from build123d import *

# Parameters (mm, degrees)
SKETCH1_W           = 50
SKETCH1_H           = 100
SKETCH1_R           = 2
SKETCH1_R_2         = 2.5
SKETCH1_W_2         = 3
SKETCH1_H_2         = 20
BOSS_EXTRUDE1_DEPTH = 3
SKETCH2_W           = 3
SKETCH2_H           = 10
CUT_EXTRUDE1_DEPTH  = 10
SKETCH3_W           = 5
SKETCH3_H           = 3
CUT_EXTRUDE2_DEPTH  = 56.982140009


with BuildPart() as part:
    # Sketch1 → Boss-Extrude1 (new body)
    with BuildSketch(Plane.XY):
        Rectangle(SKETCH1_W, SKETCH1_H)
        with Locations((-9, 44)):
            Circle(SKETCH1_R, mode=Mode.SUBTRACT)
        with Locations(Location((9, 44, 0), (0, 0, 180))):
            Circle(SKETCH1_R, mode=Mode.SUBTRACT)
        with Locations(Location((-9, 20, 0), (0, 0, 180))):
            Circle(SKETCH1_R, mode=Mode.SUBTRACT)
        with Locations((9, 20)):
            Circle(SKETCH1_R, mode=Mode.SUBTRACT)
        with Locations((-7.5, -45)):
            Circle(SKETCH1_R_2, mode=Mode.SUBTRACT)
        with Locations(Location((7.5, -45, 0), (0, 0, 180))):
            Circle(SKETCH1_R_2, mode=Mode.SUBTRACT)
        with Locations((6, -6.851771234)):
            Rectangle(SKETCH1_W_2, SKETCH1_H_2, mode=Mode.SUBTRACT)
        with Locations((-6, -6.851771234)):
            Rectangle(SKETCH1_W_2, SKETCH1_H_2, mode=Mode.SUBTRACT)
    extrude(amount=BOSS_EXTRUDE1_DEPTH)

    # Sketch2 → Cut-Extrude1 (cut)
    with BuildSketch(Plane.XY.offset(3)):
        with Locations((3.25, -25)):
            Rectangle(SKETCH2_W, SKETCH2_H)
        with Locations((-3.25, -25)):
            Rectangle(SKETCH2_W, SKETCH2_H)
    extrude(amount=-CUT_EXTRUDE1_DEPTH, mode=Mode.SUBTRACT)

    # Sketch3 → Cut-Extrude2 (cut, through all)
    with BuildSketch(Plane.XY.offset(3)):
        with Locations((-7.5, -34.709613659)):
            Rectangle(SKETCH3_W, SKETCH3_H)
        with Locations((7.5, -34.709613659)):
            Rectangle(SKETCH3_W, SKETCH3_H)
    extrude(amount=-CUT_EXTRUDE2_DEPTH, mode=Mode.SUBTRACT)


solid = part.part
Geometry: final body of the model. Coordinates: model frame, mm. A direction names the side the tool comes from. Round coordinates to 2 decimals unless told otherwise and drop trailing zeros. Order: outer loops, then holes, each group sorted by start corner. A loop starts at its lowest first (then second) coordinate and runs counter-clockwise, first axis right, second up.
Q1. Section A-A, the plane x = 9. Output: boundary loops of the cut face in (y, z).
Result sheet:
outline: (-50, 0) - (-47, 0) - (-47, 3) - (-50, 3) - close; (-43, 0) - (-36.21, 0) - (-36.21, 3) - (-43, 3) - close; (-33.21, 0) - (18, 0) - (18, 3) - (-33.21, 3) - close; (22, 0) - (42, 0) - (42, 3) - (22, 3) - close; (46, 0) - (50, 0) - (50, 3) - (46, 3) - close
Q2. Material intervals for probe 1 along X at (y, z) = (-6, 1.8); probe 2 along Y at (x, z) = (-10.5, 2.5); probe 3 along Y at (x, z) = (-9, 1.35), sorted ascending.
Result sheet:
probe 1: x = -25 to -7.5, -4.5 to 4.5, 7.5 to 25
probe 2: y = -50 to 18.68, 21.32 to 42.68, 45.32 to 50
probe 3: y = -50 to -47, -43 to -36.21, -33.21 to 18, 22 to 42, 46 to 50
Q3. Mould query, pull axis X, two halves, no side actions, for faces 3 (the face through (3, -30, 2)), 4 (the face through (-25, -1, 1)), 5 (the face through (25, -1, 1)). Classes: released by +X, released by -X, zero draft, split by the parting line, or undercut.
Result sheet:
face 3: undercut
face 4: released by -X
face 5: released by +X
Q4. Section D-D, the plane y = -11. Output: boundary loops of the cut face in (x, z).
Result sheet:
outline: (-25, 0) - (-7.5, 0) - (-7.5, 3) - (-25, 3) - close; (-4.5, 0) - (4.5, 0) - (4.5, 3) - (-4.5, 3) - close; (7.5, 0) - (25, 0) - (25, 3) - (7.5, 3) - close
Q5. Access query for faces 1 (the face through (0, -50, 1)), 2 (the face through (-6, 3.148, 1)). Directions: +Z, -Z, +X, -X, +Y, -Y. A direction counts if a zero-diameter tool reaches every point of the face in a straight line with its end or side. Return the directions, or none.
Result sheet:
face 1: +Z, -Z, +X, -X, -Y
face 2: +Z, -Z
Q6. Section C-C, the plane z = 2.55. Give the number of separate pieces and of enclosed holes in the cut face, and give its area (3 significant figures).
Result sheet:
separate pieces: 1
enclosed holes: 12
area: 4,700 mm2
Q7. Pin query (flat end, axial travel): pin 1 (3.5 mm diameter, centred on x = -9, y = 44, fed in from -Z). Return the tip coordinate at first contact, or that it passes through.
Result sheet:
pin 1: passes through
Q8. Section B-B, the plane y = -45. Output: boundary loops of the cut face in (x, z), and give its area (3 significant figures).
Result sheet:
outline: (-25, 0) - (-10, 0) - (-10, 3) - (-25, 3) - close; (-5, 0) - (5, 0) - (5, 3) - (-5, 3) - close; (10, 0) - (25, 0) - (25, 3) - (10, 3) - close
area: 120 mm2
